from build123d import *

# Parameters (mm, degrees)
BOSS_EXTRUDE1_DEPTH = 1.5


with BuildPart() as part:
    # Sketch2 → Boss-Extrude1 (new body)
    with BuildSketch(Plane.XY):
        with BuildLine():
            Line((-27.517156851, -1.370401199), (-27.517156851, 8.629598801))
            Line((-27.517156851, 8.629598801), (-22.517156851, 8.629598801))
            Line((-22.517156851, 8.629598801), (-22.517156851, 10.129598801))
            Line((-22.517156851, 10.129598801), (-17.517156851, 10.129598801))
            Line((-17.517156851, 10.129598801), (-17.517156851, 8.629598801))
            Line((-17.517156851, 8.629598801), (-12.517156851, 8.629598801))
            Line((-12.517156851, 8.629598801), (-12.517156851, 10.129598801))
            Line((-12.517156851, 10.129598801), (-7.517156851, 10.129598801))
            Line((-7.517156851, 10.129598801), (-7.517156851, 8.629598801))
            Line((-7.517156851, 8.629598801), (22.482843149, 8.629598801))
            Line((22.482843149, 8.629598801), (22.482843149, -7.370401199))
            Line((22.482843149, -7.370401199), (12.482843149, -7.370401199))
            ThreePointArc((12.482843149, -7.370401199), (5.615628068, -2.788438903), (-2.517156851, -1.370401199))
            Line((-2.517156851, -1.370401199), (-7.517156851, -1.370401199))
            Line((-7.517156851, -1.370401199), (-7.517156851, -2.870401199))
            Line((-7.517156851, -2.870401199), (-12.517156851, -2.870401199))
            Line((-12.517156851, -2.870401199), (-12.517156851, -1.370401199))
            Line((-12.517156851, -1.370401199), (-17.517156851, -1.370401199))
            Line((-17.517156851, -1.370401199), (-17.517156851, -2.870401199))
            Line((-17.517156851, -2.870401199), (-22.517156851, -2.870401199))
            Line((-22.517156851, -2.870401199), (-22.517156851, -1.370401199))
            Line((-22.517156851, -1.370401199), (-27.517156851, -1.370401199))
        make_face()
    extrude(amount=BOSS_EXTRUDE1_DEPTH)


solid = part.part
Geometry check sheet. Reference: the model listing, model coordinates, mm. A direction names the side the tool comes from. Give positions to 0.01 mm unless a question says otherwise; leave off trailing zeros. Loops run counter-clockwise (first coordinate to the right, second up) from the corner with the lowest first, then second, coordinate; pieces in that order, holes last.
(1) Thickness scan on L1, parallel to Y at x = -23, z = 0.2; L2, parallel to Y at x = -22, z = 0.6; L3, parallel to X at y = -4.75, z = 0.1. Record the ranges inside material, lowest first.
From the geometry:
L1: y = -1.37 to 8.63
L2: y = -2.87 to 10.13
L3: x = 9.33 to 22.48
(2) Set-up check for faces 1 (the flat face through (-17.517, 9, 1)), 2 (the flat face through (-22.517, 9, 1)), 3 (the flat face through (-5, -1.37, 1)), 4 (the flat face through (-20, -2.87, 1)): record each of +Z, -Z, +X, -X, +Y, -Y from which the full face is reachable in a straight line by a thin tool's end or side.
From the geometry:
face 1: +Z, -Z, +Y
face 2: +Z, -Z, -X, +Y
face 3: +Z, -Z, -Y
face 4: +Z, -Z, -X, -Y
(3) Release check for a two-part mould opening along X. For faces 5 (the flat face through (-7.517, 9, 1)), 6 (the flat face through (-12.517, -2, 1)), 7 (the flat face through (-15, 8.63, 1)), 8 (the flat face through (-10, -2.87, 1)) record: released by +X, released by -X, zero draft, split by the parting line, or undercut.
From the geometry:
face 5: released by +X
face 6: undercut
face 7: undercut
face 8: zero draft
(4) Depth check by flat-ended pin: pin 1 Ø5 at (x, y) = (11.5, 3.5) entering from -Z; pin 2 Ø0.8 at (x, z) = (-5, 0.5) entering from -Y; pin 3 Ø0.8 at (x, z) = (-25.5, 0.5) entering from +Y; pin 4 Ø0.7 at (y, z) = (-2, 0.5) entering from -X. Enter the tip coordinate at first touch or a pass-through.
From the geometry:
pin 1: stops at z = 0
pin 2: stops at y = -1.37
pin 3: stops at y = 8.63
pin 4: stops at x = -22.52
(5) Section check C-C on x = -15.5. Record the cut outline in (y, z), then the cut area to 3 significant figures.
From the geometry:
outline: (-1.37, 0) - (8.63, 0) - (8.63, 1.5) - (-1.37, 1.5) - close
area: 15.0 mm2
(6) Section check A-A on z = 0.65. Record the cut outline in (x, y), then the cut area to 3 significant figures.
From the geometry:
outline: (-27.52, -1.37) - (-22.52, -1.37) - (-22.52, -2.87) - (-17.52, -2.87) - (-17.52, -1.37) - (-12.52, -1.37) - (-12.52, -2.87) - (-7.52, -2.87) - (-7.52, -1.37) - (-2.52, -1.37) arc R20 cw to (12.48, -7.37) - (22.48, -7.37) - (22.48, 8.63) - (-7.52, 8.63) - (-7.52, 10.13) - (-12.52, 10.13) - (-12.52, 8.63) - (-17.52, 8.63) - (-17.52, 10.13) - (-22.52, 10.13) - (-22.52, 8.63) - (-27.52, 8.63) - close
area: 616 mm2
(7) Section check B-B on x = -9. Record the cut outline in (y, z).
From the geometry:
outline: (-2.87, 0) - (10.13, 0) - (10.13, 1.5) - (-2.87, 1.5) - close
